```python
from build123d import *

# Parameters (mm, degrees)
SKETCH1_W               = 100
SKETCH1_H               = 80
BOSS_EXTRUDE1_DEPTH     = 3
SKETCH2_W               = 100
SKETCH2_H               = 80
SKETCH2_W_2             = 97
SKETCH2_H_2             = 77
BOSS_EXTRUDE2_DEPTH     = 70
CUT_EXTRUDE1_DEPTH      = 3
SKETCH5_W               = 8
SKETCH5_H               = 10.304098564
SKETCH5_R               = 2
BOSS_EXTRUDE4_DEPTH     = 5
FILLET8_R               = 1
FILLET9_R               = 1
FILLET10_R              = 1
FILLET11_R              = 1
FILLET12_R              = 1
FILLET13_R              = 1
FILLET14_R              = 1
FILLET15_R              = 1
FILLET16_R              = 1
FILLET17_R              = 1
SKETCH3_R               = 1.5
CUT_EXTRUDE2_DEPTH      = 10
SKETCH7_R               = 1.5
CUT_EXTRUDE4_DEPTH      = 10
SKETCH8_R               = 2
CUT_EXTRUDE5_DEPTH      = 10
SKETCH9_W               = 20
SKETCH9_H               = 15
SKETCH9_W_2             = 8
SKETCH9_H_2             = 13
CUT_EXTRUDE7_DEPTH      = 10
LPATTERN1_COUNT         = 2
LPATTERN1_PITCH         = 50
FILLET8_OF_LPATTERN1_R  = 1
FILLET9_OF_LPATTERN1_R  = 1
FILLET10_OF_LPATTERN1_R = 1
FILLET11_OF_LPATTERN1_R = 1
FILLET12_OF_LPATTERN1_R = 1
FILLET13_OF_LPATTERN1_R = 1
FILLET14_OF_LPATTERN1_R = 1
FILLET15_OF_LPATTERN1_R = 1
FILLET16_OF_LPATTERN1_R = 1
FILLET17_OF_LPATTERN1_R = 1


with BuildPart() as part:
    # Sketch1 → Boss-Extrude1 (new body)
    with BuildSketch(Plane(origin=(0, 0, 0), x_dir=(1, 0, 0), z_dir=(0, 1, 0))):
        Rectangle(SKETCH1_W, SKETCH1_H)
    extrude(amount=BOSS_EXTRUDE1_DEPTH)

    # Sketch2 → Boss-Extrude2 (add)
    with BuildSketch(Plane(origin=(0, 3, 0), x_dir=(1, 0, 0), z_dir=(0, 1, 0))):
        Rectangle(SKETCH2_W, SKETCH2_H)
        Rectangle(SKETCH2_W_2, SKETCH2_H_2, mode=Mode.SUBTRACT)
    extrude(amount=BOSS_EXTRUDE2_DEPTH)

    # Sketch4 → Cut-Extrude1 (cut)
    with BuildSketch(Plane.XY.offset(40)):
        with BuildLine():
            Line((-38, 13), (-23, 13))
            ThreePointArc((-23, 13), (-18, 8), (-23, 3))
            Line((-23, 3), (-38, 3))
            ThreePointArc((-38, 3), (-43, 8), (-38, 13))
        make_face()
    extrude(amount=-CUT_EXTRUDE1_DEPTH, mode=Mode.SUBTRACT)

    # Sketch5 → Boss-Extrude4 (add)
    # profile 1 of 2: a face of its own
    with BuildSketch(Plane(origin=(0, 0, -40), x_dir=(-1, 0, 0), z_dir=(0, 0, -1))):
        with Locations((54, 11)):
            Rectangle(SKETCH5_W, SKETCH5_H)
        with Locations((54, 11)):
            Circle(SKETCH5_R, mode=Mode.SUBTRACT)
    # profile 2 of 2: a face of its own
    with BuildSketch(Plane(origin=(0, 0, -40), x_dir=(-1, 0, 0), z_dir=(0, 0, -1))):
        with Locations((-54, 11)):
            Rectangle(SKETCH5_W, SKETCH5_H)
        with Locations((-54, 11)):
            Circle(SKETCH5_R, mode=Mode.SUBTRACT)
    boss_extrude4 = extrude(amount=-BOSS_EXTRUDE4_DEPTH)

    # Fillet8
    fillet8_edges = [part.edges().sort_by_distance(p)[0] for p in [
        (58, 16.152049282, -37.5),
    ]]
    fillet(fillet8_edges, radius=FILLET8_R)

    # Fillet9
    fillet9_edges = [part.edges().sort_by_distance(p)[0] for p in [
        (58, 5.847950718, -37.5),
    ]]
    fillet(fillet9_edges, radius=FILLET9_R)

    # Fillet10
    fillet10_edges = [part.edges().sort_by_distance(p)[0] for p in [
        (50, 5.847950718, -37.5),
    ]]
    fillet(fillet10_edges, radius=FILLET10_R)

    # Fillet11
    fillet11_edges = [part.edges().sort_by_distance(p)[0] for p in [
        (50, 16.152049282, -37.5),
    ]]
    fillet(fillet11_edges, radius=FILLET11_R)

    # Fillet12
    fillet12_edges = [part.edges().sort_by_distance(p)[0] for p in [
        (50, 11, -35),
    ]]
    fillet(fillet12_edges, radius=FILLET12_R)

    # Fillet13
    fillet13_edges = [part.edges().sort_by_distance(p)[0] for p in [
        (-58, 5.847950718, -37.5),
    ]]
    fillet(fillet13_edges, radius=FILLET13_R)

    # Fillet14
    fillet14_edges = [part.edges().sort_by_distance(p)[0] for p in [
        (-58, 16.152049282, -37.5),
    ]]
    fillet(fillet14_edges, radius=FILLET14_R)

    # Fillet15
    fillet15_edges = [part.edges().sort_by_distance(p)[0] for p in [
        (-50, 5.847950718, -37.5),
    ]]
    fillet(fillet15_edges, radius=FILLET15_R)

    # Fillet16
    fillet16_edges = [part.edges().sort_by_distance(p)[0] for p in [
        (-50, 16.152049282, -37.5),
    ]]
    fillet(fillet16_edges, radius=FILLET16_R)

    # Fillet17
    fillet17_edges = [part.edges().sort_by_distance(p)[0] for p in [
        (-50, 11, -35),
    ]]
    fillet(fillet17_edges, radius=FILLET17_R)

    # Sketch3 → Cut-Extrude2 (cut)
    with BuildSketch(Plane(origin=(0, 3, 0), x_dir=(1, 0, 0), z_dir=(0, 1, 0))):
        with Locations(Location((-38.5, 28.5, 0), (0, 0, 270))):
            Circle(SKETCH3_R)
        with Locations(Location((-38.5, -20.5, 0), (0, 0, 270))):
            Circle(SKETCH3_R)
        with Locations(Location((19.5, 28.5, 0), (0, 0, 270))):
            Circle(SKETCH3_R)
        with Locations(Location((19.5, -20.5, 0), (0, 0, 270))):
            Circle(SKETCH3_R)
    extrude(amount=-CUT_EXTRUDE2_DEPTH, mode=Mode.SUBTRACT)

    # Sketch7 → Cut-Extrude4 (cut)
    with BuildSketch(Plane.XY.offset(40)):
        with Locations((-35, 66)):
            Circle(SKETCH7_R)
        with Locations((34, 66)):
            Circle(SKETCH7_R)
        with Locations((-35, 17)):
            Circle(SKETCH7_R)
        with Locations((34, 17)):
            Circle(SKETCH7_R)
    extrude(amount=-CUT_EXTRUDE4_DEPTH, mode=Mode.SUBTRACT)

    # Sketch8 → Cut-Extrude5 (cut)
    with BuildSketch(Plane(origin=(0, 0, -40), x_dir=(-1, 0, 0), z_dir=(0, 0, -1))):
        with Locations((-45, 65)):
            Circle(SKETCH8_R)
        with Locations((44, 65)):
            Circle(SKETCH8_R)
        with Locations((-45, 8)):
            Circle(SKETCH8_R)
        with Locations((44, 8)):
            Circle(SKETCH8_R)
    extrude(amount=-CUT_EXTRUDE5_DEPTH, mode=Mode.SUBTRACT)

    # Sketch9 → Cut-Extrude7 (cut)
    with BuildSketch(Plane(origin=(50, 0, 0), x_dir=(0, 0, -1), z_dir=(1, 0, 0))):
        with Locations((4.6, 10)):
            Rectangle(SKETCH9_W, SKETCH9_H)
        with Locations((8.475245753, 39.06044871)):
            Rectangle(SKETCH9_W_2, SKETCH9_H_2)
    extrude(amount=-CUT_EXTRUDE7_DEPTH, mode=Mode.SUBTRACT)

    # LPattern1: Boss-Extrude4 ×2
    with Locations(*[(0, i * LPATTERN1_PITCH, 0) for i in range(1, LPATTERN1_COUNT)]):
        add(boss_extrude4)

    # Fillet8 of LPattern1
    fillet8_of_lpattern1_edges = [part.edges().sort_by_distance(p)[0] for p in [
        (58, 66.152049282, -37.5),
    ]]
    fillet(fillet8_of_lpattern1_edges, radius=FILLET8_OF_LPATTERN1_R)

    # Fillet9 of LPattern1
    fillet9_of_lpattern1_edges = [part.edges().sort_by_distance(p)[0] for p in [
        (58, 55.847950718, -37.5),
    ]]
    fillet(fillet9_of_lpattern1_edges, radius=FILLET9_OF_LPATTERN1_R)

    # Fillet10 of LPattern1
    fillet10_of_lpattern1_edges = [part.edges().sort_by_distance(p)[0] for p in [
        (50, 55.847950718, -37.5),
    ]]
    fillet(fillet10_of_lpattern1_edges, radius=FILLET10_OF_LPATTERN1_R)

    # Fillet11 of LPattern1
    fillet11_of_lpattern1_edges = [part.edges().sort_by_distance(p)[0] for p in [
        (50, 66.152049282, -37.5),
    ]]
    fillet(fillet11_of_lpattern1_edges, radius=FILLET11_OF_LPATTERN1_R)

    # Fillet12 of LPattern1
    fillet12_of_lpattern1_edges = [part.edges().sort_by_distance(p)[0] for p in [
        (50, 61, -35),
    ]]
    fillet(fillet12_of_lpattern1_edges, radius=FILLET12_OF_LPATTERN1_R)

    # Fillet13 of LPattern1
    fillet13_of_lpattern1_edges = [part.edges().sort_by_distance(p)[0] for p in [
        (-58, 55.847950718, -37.5),
    ]]
    fillet(fillet13_of_lpattern1_edges, radius=FILLET13_OF_LPATTERN1_R)

    # Fillet14 of LPattern1
    fillet14_of_lpattern1_edges = [part.edges().sort_by_distance(p)[0] for p in [
        (-58, 66.152049282, -37.5),
    ]]
    fillet(fillet14_of_lpattern1_edges, radius=FILLET14_OF_LPATTERN1_R)

    # Fillet15 of LPattern1
    fillet15_of_lpattern1_edges = [part.edges().sort_by_distance(p)[0] for p in [
        (-50, 55.847950718, -37.5),
    ]]
    fillet(fillet15_of_lpattern1_edges, radius=FILLET15_OF_LPATTERN1_R)

    # Fillet16 of LPattern1
    fillet16_of_lpattern1_edges = [part.edges().sort_by_distance(p)[0] for p in [
        (-50, 66.152049282, -37.5),
    ]]
    fillet(fillet16_of_lpattern1_edges, radius=FILLET16_OF_LPATTERN1_R)

    # Fillet17 of LPattern1
    fillet17_of_lpattern1_edges = [part.edges().sort_by_distance(p)[0] for p in [
        (-50, 61, -35),
    ]]
    fillet(fillet17_of_lpattern1_edges, radius=FILLET17_OF_LPATTERN1_R)


solid = part.part
```
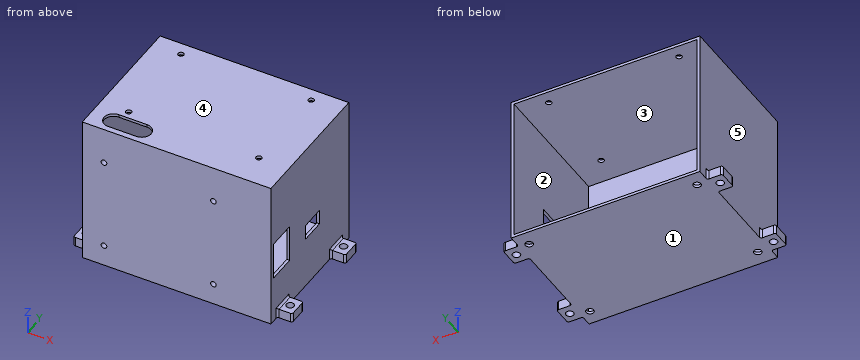
The listing builds one solid part. Answer for the finished solid, in the listing's coordinates (mm). Face numbers are marked on the shaded views. A direction names the side the tool comes from. Give positions to 0.01 mm unless a question says otherwise; leave off trailing zeros. Order: outer loops, then holes, each group sorted by start corner. A loop starts at its lowest first (then second) coordinate and runs counter-clockwise, first axis right, second up.
1) Consider line 1 along Y through (x, z) = (54, -37.25); line 2 along Z through (x, y) = (-2, 26.5); line 3 along X through (y, z) = (55.5, 16). Determine where each line is inside the solid, lowest interval first.
Reported:
line 1: y = 5.85 to 9, 13 to 16.15, 55.85 to 59, 63 to 66.15
line 2: z = -40 to -38.5, 38.5 to 40
line 3: x = -50 to -48.5, 48.5 to 50
2) Find section A-A on y = 61. Write down the section's boundary in (x, z).
Reported:
outline: (-58, -40) - (-56, -40) - (-56, -35) - (-58, -35) - close; (-52, -40) - (52, -40) - (52, -35) - (51, -35) arc R1 cw to (50, -34) - (50, 40) - (-50, 40) - (-50, -34) arc R1 cw to (-51, -35) - (-52, -35) - close; (56, -40) - (58, -40) - (58, -35) - (56, -35) - close; hole (-48.5, -38.5) - (48.5, -38.5) - (48.5, 38.5) - (-48.5, 38.5) - close
3) Given P1, Ø2, axis at x = -54.5, y = 62, coming from the +Z side; P2, Ø2, axis at y = 28, z = -11, coming from the -X side; P3, Ø1.5, axis at x = 54.5, z = -38, coming from the +Y side; P4, Ø2.5, axis at x = 19.5, z = -28.5, coming from the +Y side, each flat-ended and moving along its own axis, determine where each tip first touches the part or whether it passes through.
Reported:
P1: stops at z = -35
P2: stops at x = -50
P3: stops at y = 66.15
P4: passes through
4) Find section C-C on x = 34. Write down the section's boundary in (y, z).
Reported:
outline: (0, -40) - (73, -40) - (73, -38.5) - (3, -38.5) - (3, 38.5) - (15.5, 38.5) - (15.5, 40) - (0, 40) - close; (18.5, 38.5) - (64.5, 38.5) - (64.5, 40) - (18.5, 40) - close; (67.5, 38.5) - (73, 38.5) - (73, 40) - (67.5, 40) - close
5) Find section B-B on z = -9. Write down the section's boundary in (x, y).
Reported:
outline: (-50, 0) - (50, 0) - (50, 2.5) - (40, 2.5) - (40, 3) - (-48.5, 3) - (-48.5, 73) - (-50, 73) - close; (48.5, 17.5) - (50, 17.5) - (50, 32.56) - (48.5, 32.56) - close; (48.5, 45.56) - (50, 45.56) - (50, 73) - (48.5, 73) - close
6) For the marked faces 1 and 2, determine the directions among +Z, -Z, +X, -X, +Y, -Y from which every point of the face is accessible in a straight line to the end or side of a thin tool.
Reported:
face 1: -Z, +X, -X, +Y, -Y
face 2: +Y
7) Determine the mould class of the marked faces 3, 4 and 5 for opening direction X: pulls with the +X half, pulls with the -X half, needs draft (parallel to the pull), parting line crosses it, or undercut.
Reported:
face 3: undercut
face 4: needs draft
face 5: pulls with the -X half
8) Find section D-D on x = 54. Write down the section's boundary in (y, z), then the cut area to 3 significant figures.
Reported:
outline: (5.85, -40) - (9, -40) - (9, -35) - (5.85, -35) - close; (13, -40) - (16.15, -40) - (16.15, -35) - (13, -35) - close; (55.85, -40) - (59, -40) - (59, -35) - (55.85, -35) - close; (63, -40) - (66.15, -40) - (66.15, -35) - (63, -35) - close
area: 63.0 mm2
